Source: CAD feature listing. Evaluate the final solid. Frame: model axes, mm. Face numbers are marked on the shaded views. A direction names the side the tool comes from. Give positions to 0.01 mm unless a question says otherwise; leave off trailing zeros. Write each loop counter-clockwise with the first axis right and the second up, starting at its lowest first coordinate (ties: lowest second). Pieces come first, ordered by that corner, then holes.
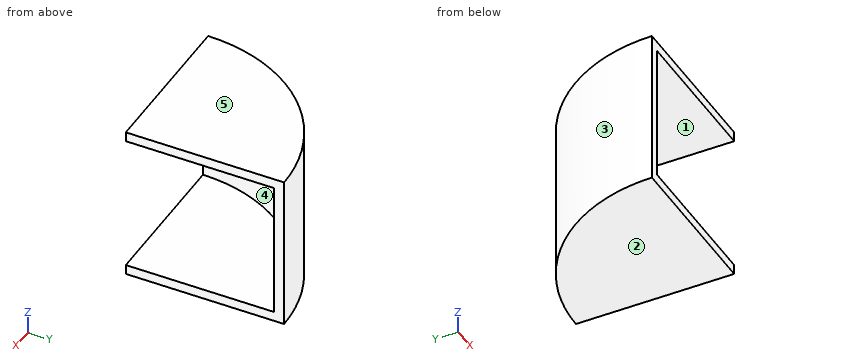
```python
from build123d import *

# Parameters (mm, degrees)
F1_DEPTH = 40
F2_T     = -2.5


with BuildPart() as f1:
    # F0 (on Top) → F1 (new body)
    with BuildSketch(Plane.XY):
        with BuildLine():
            Line((-40, 0), (0, 0))
            Line((0, 0), (0, 40))
            ThreePointArc((0, 40), (-28.284271, 28.284271), (-40, 0))
        make_face()
    extrude(amount=F1_DEPTH)

    # F2
    f2_openings = [f1.faces().sort_by_distance(p)[0] for p in [
        (-20, 0, 20),
        (0, 20, 20),
    ]]
    offset(amount=F2_T, openings=f2_openings)


solid = f1.part
```
1. Access query for the marked faces 4 and 5. Directions: +Z, -Z, +X, -X, +Y, -Y. A direction counts if a zero-diameter tool reaches every point of the face in a straight line with its end or side. Return the directions, or none.
2. Line query: probe 1 along Z at (x, y) = (-8.5, 12); probe 2 along X at (y, z) = (27, 13); probe 3 along Y at (x, z) = (-30, 9). Output: solid intervals per line, ascending.
3. Section query A-A (y = 14.5). Return loops of the section in (x, z), plus the area to 3 significant figures.
4. Section query C-C (z = 19). Return loops of the section in (x, y).
5. Section query B-B (x = -34.5). Return loops of the section in (y, z).
6. Pin query (flat end, axial travel): P1, Ø10, axis at x = -25.5, z = 22, coming from the -Y side; P2, Ø2, axis at y = 32.5, z = 23.5, coming from the +X side; P3, Ø1, axis at x = -33.5, z = 29, coming from the +Y side. Return the tip coordinate at first contact, or that it passes through.
7. Pull-direction query (Z, two-part tool) for the marked faces 1, 2 and 3; classes: pulls with the +Z half, pulls with the -Z half, needs draft (parallel to the pull), parting line crosses it, or undercut.
The answers:
1. face 4: +X, -Y
1. face 5: +Z, +X, -X, +Y, -Y
2. probe 1: z = 0 to 2.5, 37.5 to 40
2. probe 2: x = -29.51 to -26.02
2. probe 3: y = 22.5 to 26.46
3. outline: (-37.28, 0) - (0, 0) - (0, 2.5) - (-34.58, 2.5) - (-34.58, 37.5) - (0, 37.5) - (0, 40) - (-37.28, 40) - close
3. area: 281 mm2
4. outline: (-40, 0) - (-37.5, 0) arc R37.5 cw to (0, 37.5) - (0, 40) arc R40 ccw to start
5. outline: (0, 0) - (20.24, 0) - (20.24, 40) - (0, 40) - (0, 37.5) - (14.7, 37.5) - (14.7, 2.5) - (0, 2.5) - close
6. P1: stops at y = 21.82
6. P2: stops at x = -16.85
6. P3: stops at y = 22.61
7. face 1: undercut
7. face 2: pulls with the -Z half
7. face 3: needs draft
